Verification items for the finished model (mm, model axes). Give positions to 0.01 mm unless a question says otherwise; leave off trailing zeros. Order: outer loops, then holes, each group sorted by start corner. A loop starts at its lowest first (then second) coordinate and runs counter-clockwise, first axis right, second up. Notation, with made-up numbers: (61.5, -26) -> (101.5, -26) arc R27 cw to (101.5, 4) -> close; hole circle Ø5 at (23.25, 75). An arc over 180 degrees is marked (long way). Write each question's results on one line, items separated by ' | '. Start each with the question number.
1. Mould release check, pull along Z, two halves, no side actions. Record for faces 1 (the face through (-39.09, 1.61, 39.05)), 2 (the face through (-40, 2, 1)), 3 (the face through (-7.153, 1.565, 0.115)): +Z half, -Z half, draft (parallel to the pull), parting line (faces both ways), or undercut.
2. Cross-section at B-B, the plane x = 7.36. Enter the section's corners in (y, z) (3 decimals), then the cut area to 3 significant figures.
3. Material ranges on L1, parallel to X at y = 1.3, z = -0.08; L2, parallel to Z at x = -8.5, y = 0.5; L3, parallel to X at y = 2.5, z = 33.5, recorded low to high. Write a range as from..to.
4. Cross-section at C-C, the plane x = -0.64. Enter the section's corners in (y, z) (3 decimals), then the cut area to 3 significant figures.
5. Depth check by flat-ended pin: pin 1 Ø5 at (x, z) = (17, -1.5) entering from -Y. Enter the tip coordinate at first touch or a pass-through.
6. Cross-section at A-A, the plane z = -0.08. Enter the section's corners in (x, y) (3 decimals).
from build123d import *

# Parameters (mm, degrees)
SKETCH1_W           = 80
SKETCH1_H           = 80
BOSS_EXTRUDE1_DEPTH = 3.175
SKETCH16_R          = 1.984375
CUT_EXTRUDE8_DEPTH  = 10
FILLET1_R           = 3.175
SKETCH21_R          = 1.5
CUT_EXTRUDE9_DEPTH  = 10


with BuildPart() as part:
    # Sketch1 → Boss-Extrude1 (new body)
    with BuildSketch(Plane(origin=(0, 0, 0), x_dir=(1, 0, 0), z_dir=(0, 1, 0))):
        Rectangle(SKETCH1_W, SKETCH1_H)
    extrude(amount=BOSS_EXTRUDE1_DEPTH)

    # Sketch16 → Cut-Extrude8 (cut)
    with BuildSketch(Plane(origin=(0, 3.175, 0), x_dir=(1, 0, 0), z_dir=(0, 1, 0))):
        with Locations(Location((-32.800817373, 33.005763026, 0), (0, 0, 270))):
            Circle(SKETCH16_R)
        with Locations(Location((32.282136008, 32.236454615, 0), (0, 0, 270))):
            Circle(SKETCH16_R)
        with Locations(Location((31.512827597, -32.846498766, 0), (0, 0, 270))):
            Circle(SKETCH16_R)
        with Locations(Location((-33.570125785, -32.077190355, 0), (0, 0, 270))):
            Circle(SKETCH16_R)
    extrude(amount=-CUT_EXTRUDE8_DEPTH, mode=Mode.SUBTRACT)

    # Fillet1
    fillet1_edges = [part.edges().sort_by_distance(p)[0] for p in [
        (-40, 1.5875, -40),
        (40, 1.5875, -40),
        (40, 1.5875, 40),
        (-40, 1.5875, 40),
    ]]
    fillet(fillet1_edges, radius=FILLET1_R)

    # Sketch21 → Cut-Extrude9 (cut)
    with BuildSketch(Plane.XZ):
        with Locations(Location((-0.64, 7.92, 0), (0, 0, 270))):
            Circle(SKETCH21_R)
        with Locations(Location((7.36, -0.08, 0), (0, 0, 270))):
            Circle(SKETCH21_R)
        with Locations(Location((-0.64, -8.08, 0), (0, 0, 270))):
            Circle(SKETCH21_R)
        with Locations(Location((-8.64, -0.08, 0), (0, 0, 270))):
            Circle(SKETCH21_R)
    extrude(amount=-CUT_EXTRUDE9_DEPTH, mode=Mode.SUBTRACT)


solid = part.part
Results below:
1) face 1: +Z half | face 2: draft | face 3: undercut
2) outline: (0, -40) -> (3.175, -40) -> (3.175, -1.58) -> (0, -1.58) -> close; (0, 1.42) -> (3.175, 1.42) -> (3.175, 40) -> (0, 40) -> close | area: 244 mm²
3) L1: x = -40..-10.14, -7.14..5.86, 8.86..40 | L2: z = -40..-1.57, 1.41..40 | L3: x = -40..-34.95, -32.19..29.64, 33.39..40
4) outline: (0, -40) -> (3.175, -40) -> (3.175, -9.58) -> (0, -9.58) -> close; (0, -6.58) -> (3.175, -6.58) -> (3.175, 6.42) -> (0, 6.42) -> close; (0, 9.42) -> (3.175, 9.42) -> (3.175, 40) -> (0, 40) -> close | area: 235 mm²
5) pin 1: stops at y = 0
6) outline: (-40, 0) -> (-10.14, 0) -> (-10.14, 3.175) -> (-40, 3.175) -> close; (-7.14, 0) -> (5.86, 0) -> (5.86, 3.175) -> (-7.14, 3.175) -> close; (8.86, 0) -> (40, 0) -> (40, 3.175) -> (8.86, 3.175) -> close
